Autodesk Inventor part; units mm, degrees
ref_plane "YZ Plane" through (0, 0, 0) normal (1, 0, 0) x (0, 1, 0)
ref_plane "XZ Plane" through (0, 0, 0) normal (0, 1, 0) x (-1, 0, 0)
ref_plane "XY Plane" through (0, 0, 0) normal (0, 0, 1) x (1, 0, 0)
sketch "Sketch1" plane through (0, 0, 0) normal (0, 0, 1) x (1, 0, 0)
  circle A0 centre (0, 0) radius 39
  circle A1 centre (0, -27) radius 2
  circle A2 centre (23.3827, 13.5) radius 2
  circle A3 centre (-23.3827, 13.5) radius 2
  circle A4 centre (0, 0) radius 15
  dimension "d2" = 4
  dimension "d3" = 27
  dimension "d4" = 360
  dimension "d5" = 30
  dimension "d12" = 78
extrude "Extrusion1" add sketch "Sketch1" along normal blind 4
sketch "Sketch4" plane through (0, 0, 4) normal (0, 0, 1) x (1, 0, 0)
  circle A0 centre (0, 33.9) radius 1.8
  circle A1 centre (-18.3848, -8.4848) radius 1.8
  circle A2 centre (18.3848, -8.4848) radius 1.8
  circle A3 centre (0, 0) radius 39
  circle A4 centre (-23.3827, 13.5) radius 1.5001
  circle A5 centre (0, -27) radius 1.5001
  circle A6 centre (23.3827, 13.5) radius 1.5001
extrude "Extrusion4" cut sketch "Sketch4" against normal blind 4 contours A0 | A1 | A2
properties part number "SUPORT STEEP"
Read the model definition and answer for the solid it produces. Units are mm, in the model's axes. Round coordinates to 2 decimals unless told otherwise and drop trailing zeros. Write each loop counter-clockwise with the first axis right and the second up, starting at its lowest first coordinate (ties: lowest second). Pieces come first, ordered by that corner, then holes. Notation, with made-up numbers: (61.5, 33.5) - (70.5, 33.5) arc R29 cw to (70.5, 63.5) - close; hole circle Ø3 at (41, 13.5). An arc over 180 degrees is marked (long way). Use CSV: the item, a comma, the result in double quotes.
Q1. Determine the mould class of faces 1 (the cylindrical face through (-5.077, -38.668, 1.972)), 2 (the cylindrical face through (-21.475, 12.899, 1.972)), 3 (the flat face through (17, 1, 0)) for opening direction Y: +Y half, -Y half, draft (parallel to the pull), parting line (faces both ways), or undercut.
Values:
face 1,"parting line"
face 2,"undercut"
face 3,"draft"
Q2. Find section A-A, the plane y = 0. Write down the section's boundary in (x, z), then the cut area to 3 significant figures.
Values:
outline,"(-39, 0) - (-15, 0) - (-15, 4) - (-39, 4) - close; (15, 0) - (39, 0) - (39, 4) - (15, 4) - close"
area,"192 mm²"
Q3. Find section B-B, the plane x = 0. Write down the section's boundary in (y, z).
Values:
outline,"(-39, 0) - (-29, 0) - (-29, 4) - (-39, 4) - close; (-25, 0) - (-15, 0) - (-15, 4) - (-25, 4) - close; (15, 0) - (32.1, 0) - (32.1, 4) - (15, 4) - close; (35.7, 0) - (39, 0) - (39, 4) - (35.7, 4) - close"
Q4. Find section D-D, the plane y = 13.5. Write down the section's boundary in (x, z).
Values:
outline,"(-36.59, 0) - (-25.38, 0) - (-25.38, 4) - (-36.59, 4) - close; (-21.38, 0) - (-6.54, 0) - (-6.54, 4) - (-21.38, 4) - close; (6.54, 0) - (21.38, 0) - (21.38, 4) - (6.54, 4) - close; (25.38, 0) - (36.59, 0) - (36.59, 4) - (25.38, 4) - close"
Q5. Each of these flat-tipped pins is pushed along its axis until it touches: pin 1 Ø1 at (x, z) = (-28.5, 1) entering from -Y; pin 2 Ø1.5 at (y, z) = (-11.5, 3.5) entering from -X. Where does it stop, or does it pass through?
Values:
pin 1,"stops at y = -27.15"
pin 2,"stops at x = -37.49"
Q6. Straight lines are drawn through the part: line 1 along Y through (x, z) = (0, 3.2); line 2 along X through (y, z) = (-9.5, 1.7); line 3 along Y through (x, z) = (18.5, 3). For each, find the intervals that lie inside material, in ascending order.
Values:
line 1,"y = -39 to -29, -25 to -15, 15 to 32.1, 35.7 to 39"
line 2,"x = -37.83 to -19.87, -16.9 to -11.61, 11.61 to 16.9, 19.87 to 37.83"
line 3,"y = -34.33 to -10.28, -6.69 to 34.33"
Q7. Find section C-C, the plane x = 10. Write down the section's boundary in (y, z), then the cut area to 3 significant figures.
Values:
outline,"(-37.7, 0) - (-11.18, 0) - (-11.18, 4) - (-37.7, 4) - close; (11.18, 0) - (37.7, 0) - (37.7, 4) - (11.18, 4) - close"
area,"212 mm²"
